from build123d import *

# Parameters (mm, degrees)
EXTRUDE_1_DEPTH     = 3.2
SKETCH_2_R          = 12.5
SKETCH_2_R_2        = 1.6
SKETCH_2_R_3        = 1.5
SKETCH_2_R_4        = 6.45
CUT_EXTRUDE_1_DEPTH = 3.2
FILLET_1_R          = 2
FILLET_2_R          = 1


# Read off the part's stored shape, not the designer's step: 凸台-拉伸1
with BuildPart() as part:
    # 凸台-拉伸1 outline → 凸台-拉伸1 (new body)
    with BuildSketch(Plane(origin=(0, 0, 0), x_dir=(1, 0, 0), z_dir=(0, 1, 0))):
        Polygon((-55, -0.171572875), (-66.828427125, -12), (-73, -12), (-73, -30), (73, -30), (73, -12), (66.828427125, -12), (55, -0.171572875), (55, 30), (-55, 30), align=None)
        Polygon((-64, -12), (-55, -3), (-55, -12), align=None, mode=Mode.SUBTRACT)
        Polygon((55, -12), (55, -3), (64, -12), align=None, mode=Mode.SUBTRACT)
    extrude(amount=EXTRUDE_1_DEPTH)

    # 草图2 → 切除-拉伸1 (cut)
    with BuildSketch(Plane(origin=(0, 3.2, 0), x_dir=(1, 0, 0), z_dir=(0, 1, 0))):
        with Locations(Location((0, -9.443650814, 0), (0, 0, 270))):
            Circle(SKETCH_2_R)
        with Locations(Location((15.556349186, -25, 0), (0, 0, 270))):
            Circle(SKETCH_2_R_2)
        with Locations(Location((15.556349186, 6.112698372, 0), (0, 0, 270))):
            Circle(SKETCH_2_R_2)
        with Locations(Location((-15.556349186, 6.112698372, 0), (0, 0, 270))):
            Circle(SKETCH_2_R_2)
        with Locations(Location((-15.556349186, -25, 0), (0, 0, 270))):
            Circle(SKETCH_2_R_2)
        with Locations(Location((-52.5, 20, 0), (0, 0, 270))):
            Circle(SKETCH_2_R_3)
        with Locations(Location((-52.5, -20, 0), (0, 0, 270))):
            Circle(SKETCH_2_R_3)
        with Locations(Location((52.5, -20, 0), (0, 0, 270))):
            Circle(SKETCH_2_R_3)
        with Locations(Location((52.5, 20, 0), (0, 0, 270))):
            Circle(SKETCH_2_R_3)
        with Locations(Location((-64, -21, 0), (0, 0, 270))):
            Circle(SKETCH_2_R_4)
        with Locations(Location((64, -21, 0), (0, 0, 270))):
            Circle(SKETCH_2_R_4)
        with Locations(Location((42, 19, 0), (0, 0, 270))):
            Circle(SKETCH_2_R_3)
        with Locations(Location((42, 11, 0), (0, 0, 270))):
            Circle(SKETCH_2_R_3)
        with Locations(Location((-42, 11, 0), (0, 0, 270))):
            Circle(SKETCH_2_R_3)
        with Locations(Location((-42, 19, 0), (0, 0, 270))):
            Circle(SKETCH_2_R_3)
        with Locations(Location((42, -11, 0), (0, 0, 270))):
            Circle(SKETCH_2_R_3)
        with Locations(Location((42, -19, 0), (0, 0, 270))):
            Circle(SKETCH_2_R_3)
        with Locations(Location((-42, -19, 0), (0, 0, 270))):
            Circle(SKETCH_2_R_3)
        with Locations(Location((-42, -11, 0), (0, 0, 270))):
            Circle(SKETCH_2_R_3)
        with Locations(Location((-28.065, 27, 0), (0, 0, 270))):
            Circle(SKETCH_2_R_3)
        with Locations(Location((28.065, 27, 0), (0, 0, 270))):
            Circle(SKETCH_2_R_3)
        with Locations(Location((-28.065, -16.18, 0), (0, 0, 270))):
            Circle(SKETCH_2_R_3)
        with Locations(Location((28.065, -16.18, 0), (0, 0, 270))):
            Circle(SKETCH_2_R_3)
        with Locations(Location((-28.769, -27.5, 0), (0, 0, 270))):
            Circle(SKETCH_2_R_3)
        with Locations(Location((28.769, -27.5, 0), (0, 0, 270))):
            Circle(SKETCH_2_R_3)
        with Locations(Location((-36.769, -22.5, 0), (0, 0, 270))):
            Circle(SKETCH_2_R_3)
        with Locations(Location((36.769, -22.5, 0), (0, 0, 270))):
            Circle(SKETCH_2_R_3)
    extrude(amount=-CUT_EXTRUDE_1_DEPTH, mode=Mode.SUBTRACT)

    # 圆角1
    fillet_1_edges = [part.edges().sort_by_distance(p)[0] for p in [
        (-66.828427125, 1.6, 12),
        (-55, 1.6, 0.171572875),
        (-55, 1.6, -30),
        (55, 1.6, -30),
        (55, 1.6, 0.171572875),
        (66.828427125, 1.6, 12),
        (73, 1.6, 12),
        (73, 1.6, 30),
        (-73, 1.6, 30),
        (-73, 1.6, 12),
    ]]
    fillet(fillet_1_edges, radius=FILLET_1_R)

    # 圆角2
    fillet_2_edges = [part.edges().sort_by_distance(p)[0] for p in [
        (-64, 1.6, 12),
        (-55, 1.6, 12),
        (-55, 1.6, 3),
        (55, 1.6, 3),
        (55, 1.6, 12),
        (64, 1.6, 12),
    ]]
    fillet(fillet_2_edges, radius=FILLET_2_R)


solid = part.part
Could you check a few things on this model? Use its own coordinates, in mm. A direction names the side the tool comes from. Round coordinates to 2 decimals unless told otherwise and drop trailing zeros. Write each loop counter-clockwise with the first axis right and the second up, starting at its lowest first coordinate (ties: lowest second). Pieces come first, ordered by that corner, then holes. Notation, with made-up numbers: (-13, 18) - (40, 18) arc R14 ccw to (40, 36) - close; hole circle Ø2 at (21.5, 30). An arc over 180 degrees is marked (long way). Put each result on its own line as item: value. Start each with the question number.
(1) I want a section at A-A, the plane x = 10. Please give me the cut outline in (y, z).
(2) Thinking about a two-plate mould opening in X: for faces 1 (the flat face through (1, 2, -30)), 2 (the flat face through (60.99, 1.58, 6.16)), 3 (the cylindrical face through (-14.21, 1.62, -5.25)), which applies, released by +X, released by -X, zero draft, split by the parting line, or undercut?
(3) I want a section at B-B, the plane z = 16.18. Please give me the cut outline in (x, y) (3 decimals), plus the area to 3 significant figures.
(4) Will this pin go through, and if not, where does the flat tip stop? pin 1 (3 mm diameter, centred on x = 15.56, z = 25, fed in from +Y).
(5) I want a section at C-C, the plane x = 64. Please give me the cut outline in (y, z), plus the area to 3 significant figures.
(6) I want a section at D-D, the plane z = -14.5. Please give me the cut outline in (x, y).
(7) For faces 4 (the flat face through (-69, 2, 12)), 5 (the flat face through (59, 2, 12)), 6 (the flat face through (69, 2, 12)), which set-ups out of +Z, -Z, +X, -X, +Y, -Y let a thin tool reach every point of the face, with its end or its side?
(8) I need wall thicknesses on probe 1 along X at (y, z) = (2.3, -11); probe 2 along X at (y, z) = (1.55, 27.5); probe 3 along X at (y, z) = (1, -20). Which ranges of each line are inside material? Lowest first, please.
Here are the results:
1. outline: (0, -30) - (3.2, -30) - (3.2, 1.94) - (0, 1.94) - close; (0, 16.94) - (3.2, 16.94) - (3.2, 30) - (0, 30) - close
2. face 1: zero draft
2. face 2: released by +X
2. face 3: undercut
3. outline: (-73, 0) - (-68.286, 0) - (-68.286, 3.2) - (-73, 3.2) - close; (-59.714, 0) - (-29.565, 0) - (-29.565, 3.2) - (-59.714, 3.2) - close; (-26.565, 0) - (-10.53, 0) - (-10.53, 3.2) - (-26.565, 3.2) - close; (10.53, 0) - (26.565, 0) - (26.565, 3.2) - (10.53, 3.2) - close; (29.565, 0) - (59.714, 0) - (59.714, 3.2) - (29.565, 3.2) - close; (68.286, 0) - (73, 0) - (73, 3.2) - (68.286, 3.2) - close
3. area: 326 mm^2
4. pin 1: passes through
5. outline: (0, 9.17) - (3.2, 9.17) - (3.2, 14.55) - (0, 14.55) - close; (0, 27.45) - (3.2, 27.45) - (3.2, 30) - (0, 30) - close
5. area: 25.4 mm^2
6. outline: (-55, 0) - (55, 0) - (55, 3.2) - (-55, 3.2) - close
7. face 4: -Z, -X, +Y, -Y
7. face 5: +Y, -Y
7. face 6: -Z, +X, +Y, -Y
8. probe 1: x = -55 to -43.5, -40.5 to 40.5, 43.5 to 55
8. probe 2: x = -73 to -30.27, -27.27 to 27.27, 30.27 to 73
8. probe 3: x = -55 to -54, -51 to -43.12, -40.88 to 40.88, 43.12 to 51, 54 to 55
